The listing builds one solid part. Answer for the finished solid, in the listing's coordinates (mm). Round coordinates to 2 decimals unless told otherwise and drop trailing zeros. Write each loop counter-clockwise with the first axis right and the second up, starting at its lowest first coordinate (ties: lowest second). Pieces come first, ordered by that corner, then holes. Notation, with made-up numbers: M 59.5,-9.5 L 99.5,-9.5 A32 ccw 99.5,29.5 Z; hole C 54,-16 d4. An arc over 180 degrees is marked long. One line per item, written item: value. Start each with the question number.
(1) Given P1, Ø1.5, axis at x = -1, z = 86, coming from the -Y side; P2, Ø6, axis at y = 13.5, z = 31, coming from the -X side, each flat-ended and moving along its own axis, determine where each tip first touches the part or whether it passes through.
(2) Section D-D (z = 73) is taken. Determine the outline of the cut face in (x, y).
(3) Section A-A (y = 18) is taken. Determine the outline of the cut face in (x, z), plus the area to 3 significant figures.
(4) Consider probe 1 along Z at (x, y) = (-2.2, -0.5); probe 2 along Z at (x, y) = (-2.35, 8); probe 3 along Z at (x, y) = (-2.6, 24.5). Determine where each line is inside the solid, lowest interval first.
(5) Section C-C (y = 8) is taken. Determine the outline of the cut face in (x, z), plus the area to 3 significant figures.
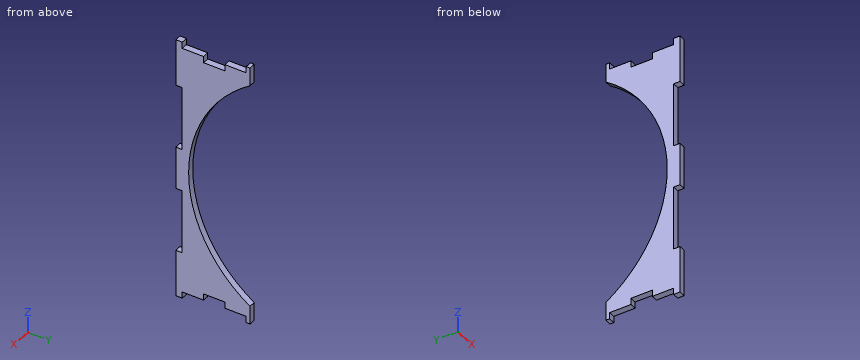
```python
from build123d import *

# Parameters (mm, degrees)
IMPORTED_START          = -3
IMPORTED_BODY_4_1_DEPTH = 3
CUT_EXTRUDE_2_DEPTH     = 3


# Read off the part's stored shape, not the designer's step: 基体零件-零件4-1
with BuildPart() as part:
    # 基体零件-零件4-1 outline → 基体零件-零件4-1 (new body)
    with BuildSketch(Plane.YZ.offset(IMPORTED_START)):
        Polygon((-3, -3), (0, -3), (0, 0), (9.999598957, 0), (9.999598957, 3), (20.000401043, 3), (20.000401043, 0), (30, 0), (30, -3), (52, -3), (52, 0), (82, 0), (82, -3), (104, -3), (104, 19), (101, 19), (101, 49), (104, 49), (104, 69), (101, 69), (101, 99), (104, 99), (104, 121), (82, 121), (82, 118), (52, 118), (52, 121), (30, 121), (30, 118), (20.000401043, 118), (20.000401043, 115), (9.999598957, 115), (9.999598957, 118), (0, 118), (0, 121), (-3, 121), (-3, 99), (0, 99), (0, 69), (-3, 69), (-3, 49), (0, 49), (0, 19), (-3, 19), align=None)
    extrude(amount=IMPORTED_BODY_4_1_DEPTH)

    # 草图3 → 切除-拉伸2 (cut)
    with BuildSketch(Plane(origin=(0, 0, 0), x_dir=(0, 0, -1), z_dir=(1, 0, 0))):
        with BuildLine():
            Line((-121, 104), (3, 104))
            Line((3, 104), (3, 31.75415679))
            Line((3, 31.75415679), (-5.579680491, 31.75415679))
            ThreePointArc((-5.579680491, 31.75415679), (-59, 3), (-112.420319509, 31.75415679))
            Line((-112.420319509, 31.75415679), (-121, 31.75415679))
            Line((-121, 31.75415679), (-121, 104))
        make_face()
    extrude(amount=-CUT_EXTRUDE_2_DEPTH, mode=Mode.SUBTRACT)


solid = part.part
```
Recorded:
1. P1: stops at y = 0
1. P2: passes through
2. outline: M -3,0 L 0,0 L 0,4.55 L -3,4.55 Z
3. outline: M -3,3 L 0,3 L 0,17.83 L -3,17.83 Z; M -3,100.17 L 0,100.17 L 0,115 L -3,115 Z
3. area: 89.0 mm2
4. probe 1: z = -3 to 19, 49 to 69, 99 to 121
4. probe 2: z = 0 to 34.2, 83.8 to 118
4. probe 3: z = 0 to 11.15, 106.85 to 118
5. outline: M -3,0 L 0,0 L 0,34.2 L -3,34.2 Z; M -3,83.8 L 0,83.8 L 0,118 L -3,118 Z
5. area: 205 mm2
